The model under review builds one solid part; all positions refer to its coordinate system, in mm. Face numbers are marked on the shaded views. A direction names the side the tool comes from. Coordinates: 2 decimals unless noted, no trailing zeros. Order: outer loops, then holes, each group sorted by start corner. A loop starts at its lowest first (then second) coordinate and runs counter-clockwise, first axis right, second up. Notation, with made-up numbers: M 39.25,73.5 L 82.25,73.5 A9 cw 82.25,90.5 Z; hole C -17,46 d10. An arc over 180 degrees is marked long. One line per item, written item: value.
```python
from build123d import *

# Parameters (mm, degrees)
SKETCH5_R           = 15.24
SKETCH6_R           = 25.4
SKETCH7_R           = 35.56
BOSS_EXTRUDE1_DEPTH = 20.32
CUT_EXTRUDE4_START  = -10.16
SKETCH8_R           = 35.56
SKETCH8_R_2         = 33.02
CUT_EXTRUDE4_DEPTH  = 10.16
SKETCH9_R           = 30.48
CUT_EXTRUDE5_DEPTH  = 17.78
SKETCH4_R           = 6.35
CUT_EXTRUDE6_DEPTH  = 118.939177545
FILLET1_R           = 2.54
BOSS_EXTRUDE2_START = 17.78
SKETCH12_R          = 30.48
BOSS_EXTRUDE2_DEPTH = 17.78
SKETCH14_R          = 6.35
CUT_EXTRUDE7_DEPTH  = 118.939177696


with BuildPart() as part:
    # Sketch3 → Revolve1 (revolve)
    with BuildSketch(Plane(origin=(0, 0, 0), x_dir=(1, 0, 0), z_dir=(0, 1, 0)), mode=Mode.PRIVATE) as revolve1_sk:
        with BuildLine():
            Line((0, 10.16), (0, -10.16))
            Line((0, -10.16), (15.24, -10.16))
            ThreePointArc((15.24, -10.16), (25.4, 0), (15.24, 10.16))
            Line((15.24, 10.16), (0, 10.16))
        make_face()
    revolve(revolve1_sk.sketch.rotate(Axis((0, 0, -50.309770133), (0, 0, 1)), 180), axis=Axis((0, 0, -50.309770133), (0, 0, 1)))

    # Sketch5 → Loft1 section 0
    with BuildSketch(Plane(origin=(0, 0, -10.16), x_dir=(-1, 0, 0), z_dir=(0, 0, -1))):
        Circle(SKETCH5_R)
    # Sketch6 → Loft1 section 1
    with BuildSketch(Plane.XY.offset(-76.2)):
        Circle(SKETCH6_R)
    loft()

    # Sketch7 → Boss-Extrude1 (add)
    with BuildSketch(Plane(origin=(0, 0, -76.2), x_dir=(-1, 0, 0), z_dir=(0, 0, -1))):
        Circle(SKETCH7_R)
    extrude(amount=BOSS_EXTRUDE1_DEPTH)

    # Sketch8 → Cut-Extrude4 (cut)
    with BuildSketch(Plane(origin=(0, 0, -91.44), x_dir=(-1, 0, 0), z_dir=(0, 0, -1)).offset(CUT_EXTRUDE4_START)):
        Circle(SKETCH8_R)
        Circle(SKETCH8_R_2, mode=Mode.SUBTRACT)
    extrude(amount=CUT_EXTRUDE4_DEPTH, mode=Mode.SUBTRACT)

    # Sketch9 → Cut-Extrude5 (cut)
    with BuildSketch(Plane(origin=(0, 0, -96.52), x_dir=(-1, 0, 0), z_dir=(0, 0, -1))):
        Circle(SKETCH9_R)
    extrude(amount=-CUT_EXTRUDE5_DEPTH, mode=Mode.SUBTRACT)

    # Sketch4 → Cut-Extrude6 (cut, through all)
    with BuildSketch(Plane.XY.offset(10.16)):
        Circle(SKETCH4_R)
    extrude(amount=-CUT_EXTRUDE6_DEPTH, mode=Mode.SUBTRACT)

    # Fillet1
    fillet1_edges = [part.edges().sort_by_distance(p)[0] for p in [
        (30.48, 0, -78.74),
    ]]
    fillet(fillet1_edges, radius=FILLET1_R)

    # Sketch12 → Boss-Extrude2 (add)
    with BuildSketch(Plane(origin=(0, 0, -78.74), x_dir=(-1, 0, 0), z_dir=(0, 0, -1)).offset(BOSS_EXTRUDE2_START)):
        Circle(SKETCH12_R)
    extrude(amount=-BOSS_EXTRUDE2_DEPTH)

    # Cut-Loft2: read off the stored shape, not the designer's step
    # Cut-Loft2: loft between two sections, ruled curve by curve
    cut_loft2_from = [
        Edge.make_bspline([(19.631934156, 16.116673394, -96.52), (-12.601412631, 55.380541707, -96.52), (-51.865280944, 23.147194919, -96.52), (-19.631934156, -16.116673394, -96.52), (12.601412631, -55.380541707, -96.52), (51.865280944, -23.147194919, -96.52), (19.631934156, 16.116673394, -96.52)], [0, 0, 0, 0, 0.5, 0.5, 0.5, 1, 1, 1, 1], 3, [1, 0.333333333, 0.333333333, 1, 0.333333333, 0.333333333, 1]),
    ]
    cut_loft2_to = [
        Edge.make_bspline([(-6.35, 0, -78.74), (-6.35, -12.7, -78.74), (6.35, -12.7, -78.74), (6.35, 0, -78.74), (6.35, 12.7, -78.74), (-6.35, 12.7, -78.74), (-6.35, 0, -78.74)], [0, 0, 0, 0, 0.5, 0.5, 0.5, 1, 1, 1, 1], 3, [1, 0.333333333, 0.333333333, 1, 0.333333333, 0.333333333, 1]),
    ]
    cut_loft2 = Solid(Shell([*[Face.make_surface_from_curves(cut_loft2_from[k], cut_loft2_to[k]) for k in range(1)], Face(Wire(cut_loft2_from)), Face(Wire(cut_loft2_to))]))
    add(cut_loft2, mode=Mode.SUBTRACT)

    # Sketch14 → Cut-Extrude7 (cut, through all)
    with BuildSketch(Plane.XY.offset(10.16)):
        Circle(SKETCH14_R)
    extrude(amount=-CUT_EXTRUDE7_DEPTH, mode=Mode.SUBTRACT)


solid = part.part
```
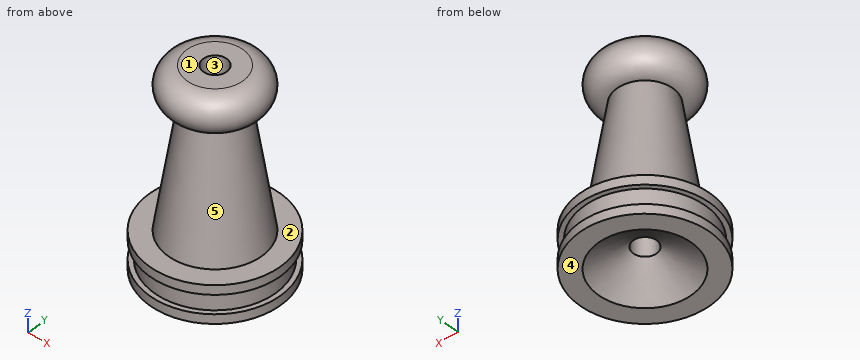
(1) We need section A-A, the plane z = -39.5. State the section outline as (x, y) points, plus the area to 3 significant figures.
Geometry results:
outline: C 0,0 d39.51; hole C 0,0 d12.7
area: 1,100 mm2
(2) Tool access review of the marked faces 1 and 2: name each direction out of +Z, -Z, +X, -X, +Y, -Y from which nothing blocks a thin tool from reaching the whole face with its end or side.
Geometry results:
face 1: +Z, +X, -X, +Y, -Y
face 2: +Z
(3) For L1, parallel to Z at x = -21, y = 25; L2, parallel to Y at x = 0, z = -11; L3, parallel to Y at x = 2, z = -88, list the stretches that pass through material, from the lowest coordinate up.
Geometry results:
L1: z = -96.52 to -76.2
L2: y = -15.37 to -6.35, 6.35 to 15.37
L3: y = -32.96 to -10.86, 10.86 to 32.96
(4) Insertion check: pin 1 Ø2 at (x, y) = (19.5, -5.5) entering from -Z; pin 2 Ø5 at (x, z) = (7, -19) entering from +Y; pin 3 Ø12 at (x, y) = (-8, 22) entering from +Z; pin 4 Ø1.5 at (x, z) = (21, -37.5) entering from +Y. Each pin has a flat end and moves straight along its axis. Give the tip position at first contact, or say it passes through.
Geometry results:
pin 1: stops at z = -94.09
pin 2: stops at y = 16.08
pin 3: stops at z = 9.93
pin 4: passes through
(5) Mouldability with a two-part tool opening along X and no side actions: class the marked faces 3, 4 and 5 as +X half, -X half, draft (parallel to the pull), parting line (faces both ways), or undercut.
Geometry results:
face 3: undercut
face 4: draft
face 5: parting line
(6) We need section B-B, the plane z = -23. State the section outline as (x, y) points.
Geometry results:
outline: C 0,0 d34.43; hole C 0,0 d12.7
